For this review, take the finished solid that the model builds, in its own axes (mm). Face numbers are marked on the shaded views. A direction names the side the tool comes from. Coordinates: 2 decimals unless noted, no trailing zeros. Loops run counter-clockwise (first coordinate to the right, second up) from the corner with the lowest first, then second, coordinate; pieces in that order, holes last. Notation, with made-up numbers: (-4, 60) - (12, 60) arc R20 ccw to (12, 95) - close; hole circle Ø2 at (52.25, 51.5). An arc over 180 degrees is marked (long way). Use one line per item in the form item = value. Start each with the question number.
1. To check wall thickness, follow probe 1 along Y at (x, z) = (5, -2); probe 2 along X at (y, z) = (4, 35); probe 3 along Y at (x, z) = (22, -17.1). State the ranges of each line that lie inside material, in increasing order.
2. Machinability: for the marked faces 1, 2 and 3, which of the approach directions +Z, -Z, +X, -X, +Y, -Y give a long, thin tool a straight path to every point of the face, cutting with its end or side? Answer none if there is none.
3. Draft analysis for pull direction Y (two halves, no side actions). For the marked faces 4, 5, 6 and 7, state which applies: +Y half, -Y half, draft (parallel to the pull), parting line (faces both ways), or undercut.
4. For pin 1 Ø0.5 at (x, z) = (87, -3.5) entering from +Y; pin 2 Ø9 at (y, z) = (13.5, -5) entering from +X; pin 3 Ø10 at (y, z) = (4.5, 8) entering from +X; pin 4 Ø12 at (x, y) = (26.5, 12) entering from +Z, all flat-tipped, find the tip position at first contact; note any pin that passes through.
5. Add section B-B on x = 5. Give the boundary of the cut face in (y, z), and give its area (3 significant figures).
6. Add section C-C on z = 32.5. Give the boundary of the cut face in (x, y).
7. Add section A-A on y = -41. Give the boundary of the cut face in (x, z).
8. Add section D-D on y = -24.5. Give the boundary of the cut face in (x, z).
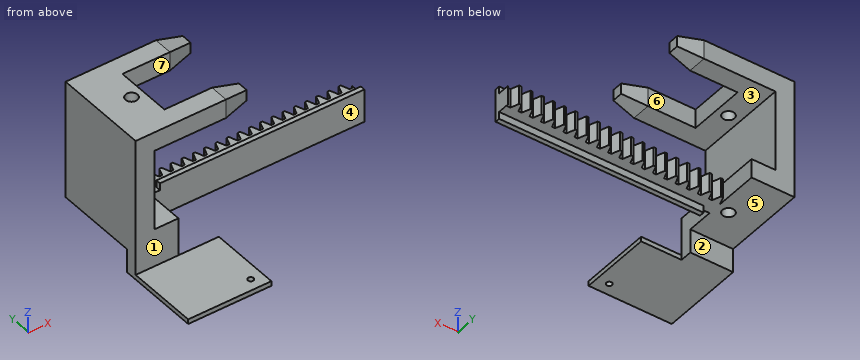
```python
from build123d import *

# Parameters (mm, degrees)
BLANKSKE_W              = 100
BLANKSKE_H              = 9.5
BLANK_DEPTH             = 8
TOOTHCUTSIM_DEPTH       = 101.768298586
TEETHCUTS_COUNT         = 22
TEETHCUTS_PITCH         = 4.712388975
SKETCH1_W               = 3
SKETCH1_H               = 2
BOSS_EXTRUDE1_DEPTH     = 100
SKETCH4_W               = 50
SKETCH4_H               = 40
BOSS_EXTRUDE2_DEPTH     = 8
SKETCH5_W               = 8
SKETCH5_H               = 8
BOSS_EXTRUDE3_DEPTH     = 30
SKETCH6_W               = 8
SKETCH6_H               = 8
BOSS_EXTRUDE4_DEPTH     = 10
BOSS_EXTRUDE4_TAPER     = 10
SKETCH7_W               = 10
SKETCH7_H               = 24
EXTRUDE_THIN1_DEPTH     = 8
SKETCH8_W               = 10
SKETCH8_H               = 40
BOSS_EXTRUDE5_DEPTH     = 8
CUT_EXTRUDE1_REACH      = 112.671
SKETCH9_W               = 14
SKETCH9_H               = 3
CUT_EXTRUDE2_DEPTH      = 116.693560775
CUT_EXTRUDE2_DEPTH_BACK = 116.693560775
SKETCH10_R              = 2.5
SKETCH11_W              = 18
SKETCH11_H              = 5
BOSS_EXTRUDE6_DEPTH     = 10
SKETCH12_W              = 35
SKETCH12_H              = 2
BOSS_EXTRUDE7_DEPTH     = 30
CUT_EXTRUDE3_REACH      = 126.419
SKETCH13_R              = 1.18


with BuildPart() as part:
    # BlankSke → Blank (new body)
    with BuildSketch(Plane.XY):
        with Locations((50, 4.75)):
            Rectangle(BLANKSKE_W, BLANKSKE_H)
    extrude(amount=-BLANK_DEPTH)

    # TooCutSkeSim → ToothCutSim (cut, through all)
    with BuildSketch(Plane.XY):
        Polygon((0.654653055, 6.125), (-0.654653055, 6.125), (-1.892297439, 9.5254), (1.892297439, 9.5254), align=None)
    toothcutsim = extrude(amount=-TOOTHCUTSIM_DEPTH, mode=Mode.SUBTRACT)

    # TeethCuts: ToothCutSim ×22
    with Locations(*[(i * TEETHCUTS_PITCH, 0, 0) for i in range(1, TEETHCUTS_COUNT)]):
        add(toothcutsim, mode=Mode.SUBTRACT)

    # Sketch1 → Boss-Extrude1 (add)
    with BuildSketch(Plane.ZY):
        with Locations((1.5, 1)):
            Rectangle(SKETCH1_W, SKETCH1_H)
    boss_extrude1 = extrude(amount=-BOSS_EXTRUDE1_DEPTH)

    # Mirror1: Boss-Extrude1 across plane
    add(boss_extrude1.mirror(Plane(origin=(0, 0, -4), x_dir=(1, 0, 0), z_dir=(0, 0, -1))))

    # Sketch4 → Boss-Extrude2 (add)
    with BuildSketch(Plane.ZY):
        with Locations((17, 4)):
            Rectangle(SKETCH4_W, SKETCH4_H)
    extrude(amount=BOSS_EXTRUDE2_DEPTH)

    # Sketch5 → Boss-Extrude3 (add)
    with BuildSketch(Plane(origin=(0, 0, 0), x_dir=(0, 0, -1), z_dir=(1, 0, 0))):
        with Locations((-38, 20)):
            Rectangle(SKETCH5_W, SKETCH5_H)
    boss_extrude3 = extrude(amount=BOSS_EXTRUDE3_DEPTH)

    # Mirror2: Boss-Extrude3 across plane
    add(boss_extrude3.mirror(Plane.ZX.offset(4)))

    # Sketch6 → Boss-Extrude4 (add)
    with BuildSketch(Plane(origin=(30, 0, 0), x_dir=(0, 0, -1), z_dir=(1, 0, 0))):
        with Locations((-38, 20)):
            Rectangle(SKETCH6_W, SKETCH6_H)
    boss_extrude4 = extrude(amount=BOSS_EXTRUDE4_DEPTH, taper=BOSS_EXTRUDE4_TAPER)

    # Mirror3: Boss-Extrude4 across plane
    add(boss_extrude4.mirror(Plane.ZX.offset(4)))

    # Sketch7 → Extrude-Thin1 (add)
    with BuildSketch(Plane.XY.offset(42)):
        with Locations((5, 4)):
            Rectangle(SKETCH7_W, SKETCH7_H)
    extrude(amount=-EXTRUDE_THIN1_DEPTH)

    # Sketch8 → Boss-Extrude5 (add)
    with BuildSketch(Plane(origin=(0, 0, -8), x_dir=(-1, 0, 0), z_dir=(0, 0, -1))):
        with Locations((-5, 4)):
            Rectangle(SKETCH8_W, SKETCH8_H)
    extrude(amount=-BOSS_EXTRUDE5_DEPTH)

    # Sketch9 → Cut-Extrude1 (cut, up to next)
    with BuildSketch(Plane(origin=(0, 2, 0), x_dir=(1, 0, 0), z_dir=(0, 1, 0)), mode=Mode.PRIVATE) as cut_extrude1_sk1:
        with Locations((7, -1.5)):
            Rectangle(SKETCH9_W, SKETCH9_H)
    cut_extrude1_tool1 = extrude(cut_extrude1_sk1.sketch, amount=-CUT_EXTRUDE1_REACH, mode=Mode.PRIVATE) & part.part
    cut_extrude1 = cut_extrude1_tool1.solids().sort_by_distance((7, 2, 1.5))[0]
    add(cut_extrude1, mode=Mode.SUBTRACT)

    # Sketch10 → Cut-Extrude2 (cut, two sides: drawn at the far end of the back side and taken through both)
    with BuildSketch(Plane.XY.offset(42).offset(-CUT_EXTRUDE2_DEPTH_BACK)):
        with Locations((5, 4)):
            Circle(SKETCH10_R)
    extrude(amount=CUT_EXTRUDE2_DEPTH + CUT_EXTRUDE2_DEPTH_BACK, mode=Mode.SUBTRACT)

    # Mirror4: Cut-Extrude1 across plane
    add(cut_extrude1.mirror(Plane(origin=(0, 0, -4), x_dir=(1, 0, 0), z_dir=(0, 0, -1))), mode=Mode.SUBTRACT)

    # Sketch11 → Boss-Extrude6 (add)
    with BuildSketch(Plane(origin=(0, 0, -8), x_dir=(-1, 0, 0), z_dir=(0, 0, -1))):
        with Locations((-1, -13.5)):
            Rectangle(SKETCH11_W, SKETCH11_H)
    extrude(amount=BOSS_EXTRUDE6_DEPTH)

    # Sketch12 → Boss-Extrude7 (add)
    with BuildSketch(Plane(origin=(0, -16, 0), x_dir=(-1, 0, 0), z_dir=(0, -1, 0))):
        with Locations((-9.5, 17)):
            Rectangle(SKETCH12_W, SKETCH12_H)
    extrude(amount=BOSS_EXTRUDE7_DEPTH)

    # Sketch13 → Cut-Extrude3 (cut, up to next)
    with BuildSketch(Plane.XY.offset(-16), mode=Mode.PRIVATE) as cut_extrude3_sk1:
        with Locations((22, -41)):
            Circle(SKETCH13_R)
    cut_extrude3_tool1 = extrude(cut_extrude3_sk1.sketch, amount=-CUT_EXTRUDE3_REACH, mode=Mode.PRIVATE) & part.part
    add(cut_extrude3_tool1.solids().sort_by_distance((22, -41, -16))[0], mode=Mode.SUBTRACT)


solid = part.part
```
Conclusion:
q1.probe_1 = -16 to 1.5, 6.5 to 24
q1.probe_2 = -8 to 2.5, 7.5 to 10
q1.probe_3 = -46 to -42.18, -39.82 to -16
q2.face_1 = +Z, +X, -X, -Y
q2.face_2 = -Z, +X, -X, +Y
q2.face_3 = +X, +Y, -Y
q3.face_4 = -Y half
q3.face_5 = draft
q3.face_6 = undercut
q3.face_7 = undercut
q4.pin_1 = 9.5
q4.pin_2 = 97.26
q4.pin_3 = 0
q4.pin_4 = 42
q5.outline = (-46, -18) - (-11, -18) - (-11, -8) - (1.5, -8) - (1.5, 0) - (-16, 0) - (-16, -16) - (-46, -16) - close; (-16, 34) - (1.5, 34) - (1.5, 42) - (-16, 42) - close; (6.5, -8) - (24, -8) - (24, 0) - (6.5, 0) - close; (6.5, 34) - (24, 34) - (24, 42) - (6.5, 42) - close
q5.area = 670 mm^2
q6.outline = (-8, -16) - (0, -16) - (0, 24) - (-8, 24) - close
q7.outline = (-8, -18) - (20.82, -18) - (20.82, -16) - (-8, -16) - close; (23.18, -18) - (27, -18) - (27, -16) - (23.18, -16) - close
q8.outline = (-8, -18) - (27, -18) - (27, -16) - (-8, -16) - close
